Answer from the drawing. Dimensions are ordinates in mm from the lowest x, y and z of the part. A direction names the side the tool comes from. Coordinates: 2 decimals unless noted, no trailing zeros. Order: outer loops, then holes, each group sorted by start corner. A loop starts at its lowest first (then second) coordinate and runs counter-clockwise, first axis right, second up. Notation, with made-up numbers: (18.25, 16) -> (75.25, 16) arc R25 ccw to (75.25, 39) -> close; hole circle Ø4 at (32, -3.5). An arc over 180 degrees is marked (long way). Answer as a JSON object with one key per item and string values. Group by question number.
1) Section C-C on x = 1.5 is taken. Determine the outline of the cut face in (y, z), and give its area (3 significant figures).
2) Section A-A on z = 5 is taken. Determine the outline of the cut face in (x, y), and give its area (3 significant figures).
3) A tool of negligible diameter and unlimited length cuts with its end or side. For the marked faces 1 and 2, from which of +Z, -Z, +X, -X, +Y, -Y can it reach the whole face along a straight path? Write none if from no direction.
4) Determine the mould class of the marked faces 3, 4 and 5 for opening direction X: released by +X, released by -X, zero draft, split by the parting line, or undercut.
5) Section D-D on y = 1.5 is taken. Determine the outline of the cut face in (x, z), and give its area (3 significant figures).
6) Section B-B on y = 3.5 is taken. Determine the outline of the cut face in (x, z), and give its area (3 significant figures).
7) Consider L1, parallel to Y at x = 2, z = 5; L2, parallel to X at y = 0.5, z = 6.5; L3, parallel to Z at x = 6.75, y = 6. Determine where each line is inside the solid, lowest interval first.
8) Given pin 1 (4 mm diameter, centred on x = 7, z = 6, fed in from +Y); pin 2 (3 mm diameter, centred on x = 4.5, y = 7, fed in from -Z); pin 3 (3 mm diameter, centred on x = 4, y = 7.5, fed in from +Z); pin 4 (1.5 mm diameter, centred on y = 4, z = 5, fed in from -X), each flat-ended and moving along its own axis, determine where each tip first touches the part or whether it passes through.
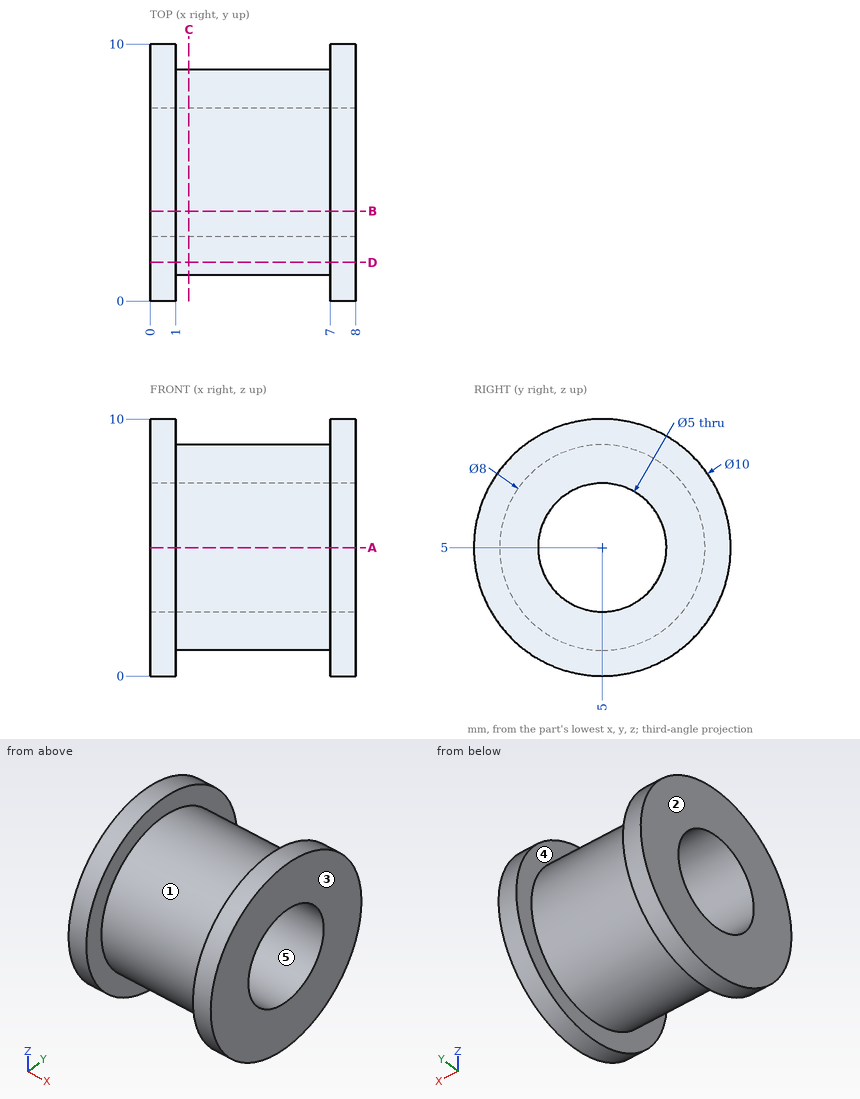
Worked answers:
{
 "1": {"outline": "circle Ø8 at (5, 5); hole circle Ø5 at (5, 5)", "area": "30.6 mm²"},
 "2": {"outline": "(0, 0) -> (1, 0) -> (1, 1) -> (7, 1) -> (7, 0) -> (8, 0) -> (8, 2.5) -> (0, 2.5) -> close; (0, 7.5) -> (8, 7.5) -> (8, 10) -> (7, 10) -> (7, 9) -> (1, 9) -> (1, 10) -> (0, 10) -> close", "area": "28.0 mm²"},
 "3": {"face 1": "none", "face 2": "+Z, -Z, -X, +Y, -Y"},
 "4": {"face 3": "released by +X", "face 4": "undercut", "face 5": "zero draft"},
 "5": {"outline": "(0, 1.43) -> (1, 1.43) -> (1, 3.06) -> (7, 3.06) -> (7, 1.43) -> (8, 1.43) -> (8, 8.57) -> (7, 8.57) -> (7, 6.94) -> (1, 6.94) -> (1, 8.57) -> (0, 8.57) -> close", "area": "37.5 mm²"},
 "6": {"outline": "(0, 0.23) -> (1, 0.23) -> (1, 1.29) -> (7, 1.29) -> (7, 0.23) -> (8, 0.23) -> (8, 3) -> (0, 3) -> close; (0, 7) -> (8, 7) -> (8, 9.77) -> (7, 9.77) -> (7, 8.71) -> (1, 8.71) -> (1, 9.77) -> (0, 9.77) -> close", "area": "31.6 mm²"},
 "7": {"L1": "y = 1 to 2.5, 7.5 to 9", "L2": "x = 0 to 1, 7 to 8", "L3": "z = 1.13 to 2.71, 7.29 to 8.87"},
 "8": {"pin 1": "stops at y = 10", "pin 2": "stops at z = 1.03", "pin 3": "stops at z = 8.87", "pin 4": "passes through"}
}
